Check sheet for the modelled part. Datum: model origin and axes. Units: mm. Face numbers are marked on the shaded views. A direction names the side the tool comes from. Coordinates: 2 decimals unless noted, no trailing zeros. Loops run counter-clockwise (first coordinate to the right, second up) from the corner with the lowest first, then second, coordinate; pieces in that order, holes last. Notation, with made-up numbers: (68.25, 34) -> (109.25, 34) arc R24 cw to (109.25, 73) -> close; hole circle Ø8 at (33.25, 62.25). An arc over 180 degrees is marked (long way). Use CSV: the item, a comma, the result in double quotes. Start each with the question number.
1. Sectioned sample at A-A, the plane z = 0. Record the cut outline in (x, y), and give its area (3 significant figures).
2. Sectioned sample at C-C, the plane z = -16.5. Record the cut outline in (x, y), and give its area (3 significant figures).
3. Sectioned sample at B-B, the plane x = -9.5. Record the cut outline in (y, z), and give its area (3 significant figures).
4. Release check for a two-part mould opening along Y. For the marked faces 1, 2, 3 and 4 record: pulls with the +Y half, pulls with the -Y half, needs draft (parallel to the pull), parting line crosses it, or undercut.
5. Thickness scan on L1, parallel to Y at x = 10, z = 0; L2, parallel to Z at x = -5, y = 0.5; L3, parallel to Z at x = 1.5, y = 0. Record the ranges inside material, lowest first.
6. Gauge pin test, flat ends, axial feed: pin 1 (1.5 mm diameter, centred on x = -16, y = 6, fed in from +Z); pin 2 (1 mm diameter, centred on x = -9.5, y = 12, fed in from -Z); pin 3 (1 mm diameter, centred on x = -10.5, z = -2, fed in from +Y); pin 4 (1.5 mm diameter, centred on x = -17.5, z = 14.5, fed in from +Y). Record the tip position at first contact, or that the pin passes through.
7. Set-up check for the marked faces 5, 6 and 7: record each of +Z, -Z, +X, -X, +Y, -Y from which the full face is reachable in a straight line by a thin tool's end or side.
```python
from build123d import *

# Parameters (mm, degrees)
F2_SIZE2 = 3
F2_SIZE  = 1.7320508076
F3_R     = 8.7
F4_DEPTH = 4.5


with BuildPart() as f1:
    # F0 (on Front) → F1 (revolve)
    with BuildSketch(Plane.XZ):
        Polygon((-23.5, 8.7), (23.5, 8.7), (23.5, 13.2), (7.5, 13.2), (7.5, 15.7), (-7.5, 15.7), (-7.5, 13.2), (-23.5, 13.2), align=None)
    revolve(axis=Axis((-11.75, 0, 0), (1, 0, 0)))

    # F2
    f2_edges = [f1.edges().sort_by_distance(p)[0] for p in [
        (23.5, 0, -8.7),
        (-23.5, 0, -8.7),
    ]]
    f2_side = f1.faces().sort_by_distance((0, 0, -8.7))[0]
    chamfer(f2_edges, length=F2_SIZE, length2=F2_SIZE2, reference=f2_side)

    # F3 (on Right) → F4 (join, symmetric)
    with BuildSketch(Plane.YZ):
        Polygon((17, -9.8149545762), (17, 9.8149545762), (0, 19.6299091524), (-17, 9.8149545762), (-17, -9.8149545762), (0, -19.6299091524), align=None)
        Circle(F3_R, mode=Mode.SUBTRACT)
    extrude(amount=F4_DEPTH, both=True)


solid = f1.part
```
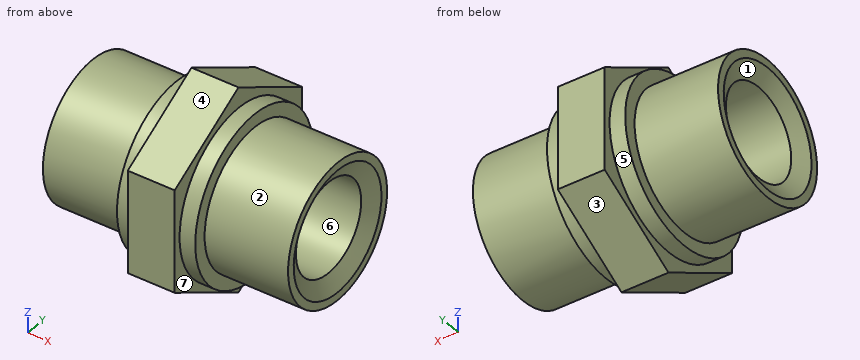
Completed:
1,outline,"(-23.5, -13.2) -> (-7.5, -13.2) -> (-7.5, -15.7) -> (-4.5, -15.7) -> (-4.5, -17) -> (4.5, -17) -> (4.5, -15.7) -> (7.5, -15.7) -> (7.5, -13.2) -> (23.5, -13.2) -> (23.5, -11.7) -> (21.77, -8.7) -> (-21.77, -8.7) -> (-23.5, -11.7) -> close; (-23.5, 11.7) -> (-21.77, 8.7) -> (21.77, 8.7) -> (23.5, 11.7) -> (23.5, 13.2) -> (7.5, 13.2) -> (7.5, 15.7) -> (4.5, 15.7) -> (4.5, 17) -> (-4.5, 17) -> (-4.5, 15.7) -> (-7.5, 15.7) -> (-7.5, 13.2) -> (-23.5, 13.2) -> close"
1,area,"511 mm²"
2,outline,"(-4.5, -5.42) -> (4.5, -5.42) -> (4.5, 5.42) -> (-4.5, 5.42) -> close"
2,area,"97.6 mm²"
3,outline,"circle Ø26.4 at (0, 0); hole circle Ø17.4 at (0, 0)"
3,area,"310 mm²"
4,face 1,"undercut"
4,face 2,"parting line crosses it"
4,face 3,"pulls with the +Y half"
4,face 4,"pulls with the -Y half"
5,L1,"-13.2 to -8.7, 8.7 to 13.2"
5,L2,"-15.69 to -8.69, 8.69 to 15.69"
5,L3,"-19.63 to -8.7, 8.7 to 19.63"
6,pin 1,"z = 12.11"
6,pin 2,"z = -6.48"
6,pin 3,"y = 13.11"
6,pin 4,"through"
7,face 5,"-X"
7,face 6,"+X, -X"
7,face 7,"+X"
